Autodesk Inventor part; units mm, degrees
ref_plane "YZ Plane" through (0, 0, 0) normal (1, 0, 0) x (0, 1, 0)
ref_plane "XZ Plane" through (0, 0, 0) normal (0, 1, 0) x (-1, 0, 0)
ref_plane "XY Plane" through (0, 0, 0) normal (0, 0, 1) x (1, 0, 0)
sketch "Sketch1" plane through (0, 0, 0) normal (0, 0, 1) x (1, 0, 0)
  line L0 (0, 0) -> (38.1, 0)
  line L1 (38.1, 0) -> (38.1, 3.175)
  line L2 (38.1, 3.175) -> (0, 3.175)
  line L3 (0, 3.175) -> (0, 0)
  dimension "d0" = 38.1
  dimension "d1" = 3.175
extrude "Extrusion1" add sketch "Sketch1" along normal blind 355.6
sketch "Sketch2" plane through (0, 0, 355.6) normal (0, 0, 1) x (1, 0, 0)
  line L0 (0, 0) -> (3.175, 0)
  line L1 (3.175, 0) -> (3.175, 38.1)
  line L2 (3.175, 38.1) -> (0, 38.1)
  line L3 (0, 38.1) -> (0, 0)
  dimension "d4" = 3.175
  dimension "d5" = 38.1
extrude "Extrusion2" add sketch "Sketch2" against normal blind 355.6
sketch "Sketch3" plane through (3.175, 38.1, 355.6) normal (0, 1, 0) x (1, 0, 0)
  line L0 (-3.175, 355.6) -> (0, 355.6)
  line L1 (0, 355.6) -> (0, 0)
  line L2 (0, 0) -> (-3.175, 0)
  line L3 (-3.175, 0) -> (-3.175, 355.6)
extrude "Extrusion3" add sketch "Sketch3" along normal blind 12.7
sketch "Sketch4" plane through (38.1, 3.175, 355.6) normal (1, 0, 0) x (0, 0, -1)
  line L0 (355.6, -3.175) -> (0, -3.175)
  line L1 (0, -3.175) -> (0, 0)
  line L2 (0, 0) -> (355.6, 0)
  line L3 (355.6, 0) -> (355.6, -3.175)
extrude "Extrusion4" add sketch "Sketch4" along normal blind 12.7
properties part number "14in 2inL Channel"
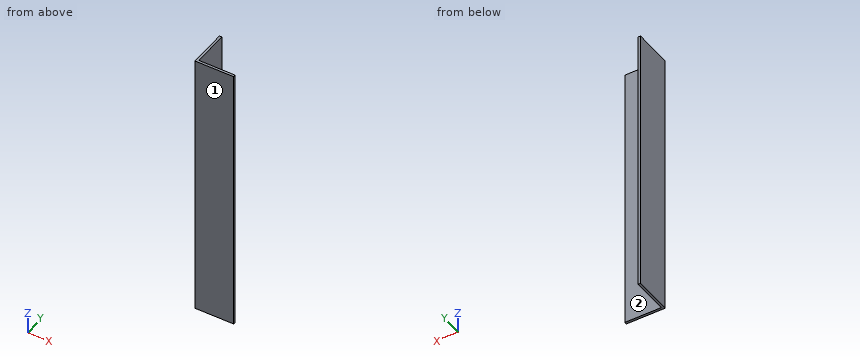
Verification items for the finished model (mm, model axes). Face numbers are marked on the shaded views. A direction names the side the tool comes from. Give positions to 0.01 mm unless a question says otherwise; leave off trailing zeros. Loops run counter-clockwise (first coordinate to the right, second up) from the corner with the lowest first, then second, coordinate; pieces in that order, holes last.
1) Set-up check for the marked faces 1 and 2: record each of +Z, -Z, +X, -X, +Y, -Y from which the full face is reachable in a straight line by a thin tool's end or side.
2) Sectioned sample at A-A, the plane z = 71. Enter the section's corners in (x, y) (3 decimals).
3) Thickness scan on line 1 along Y through (x, z) = (20, 211.5) (3 decimals). Record the ranges inside material, lowest first.
4) Depth check by flat-ended pin: pin 1 Ø3 at (x, z) = (39, 280.5) entering from +Y (3 decimals); pin 2 Ø24 at (y, z) = (33.5, 195) entering from +X (3 decimals); pin 3 Ø1.5 at (x, z) = (9, 266) entering from -Y. Enter the tip coordinate at first touch or a pass-through.
5) Sectioned sample at B-B, the plane x = 12. Enter the section's corners in (y, z) (3 decimals).
Answers:
1. face 1: +Z, -Z, +X, -X, -Y
1. face 2: +Z, -Z, +X, +Y
2. outline: (0, 0) - (50.8, 0) - (50.8, 3.175) - (3.175, 3.175) - (3.175, 50.8) - (0, 50.8) - close
3. line 1: y = 0 to 3.175
4. pin 1: stops at y = 3.175
4. pin 2: stops at x = 3.175
4. pin 3: stops at y = 0
5. outline: (0, 0) - (3.175, 0) - (3.175, 355.6) - (0, 355.6) - close
